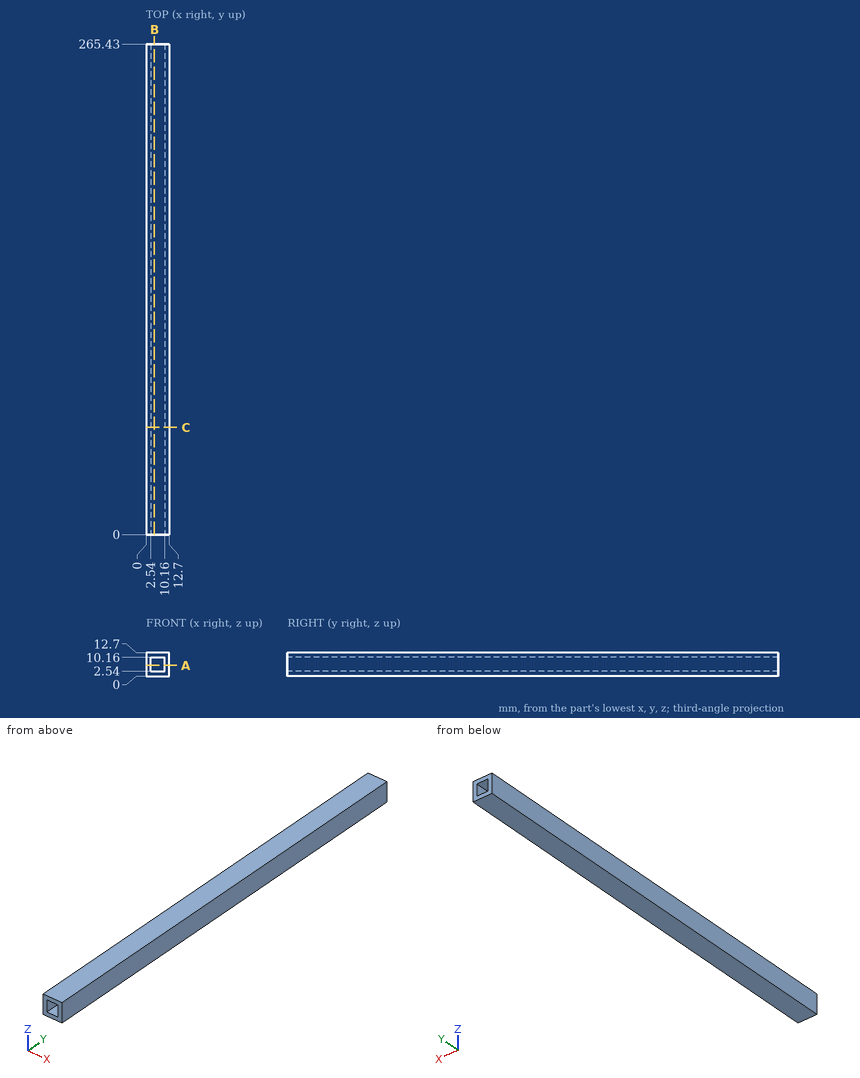
The drawing under review shows one solid part. Ordinate dimensions are in mm from its lowest x, y, z. Coordinates: 2 decimals unless noted, no trailing zeros. Order: outer loops, then holes, each group sorted by start corner. A loop starts at its lowest first (then second) coordinate and runs counter-clockwise, first axis right, second up. Notation, with made-up numbers: (45.5, -19) -> (71.5, -19) arc R19 ccw to (71.5, 13) -> close; hole circle Ø11 at (50, 9). An arc over 180 degrees is marked (long way). Answer in a Markdown table with one row per item. Add a question column.
Item 1: We need section A-A on z = 5.75. Write out the cut boundary in (x, y).
Item 2: We need section C-C on y = 58. Write out the cut boundary in (x, z), plus the area to 3 significant figures.
Item 3: To check wall thickness, follow probe 1 along X at (y, z) = (126, 7.75). State the ranges of the line that lie inside material, in increasing order.
Item 4: We need section B-B on x = 4.5. Write out the cut boundary in (y, z), plus the area to 3 significant figures.
Final values:
| question | item | result |
|---|---|---|
| 1 | outline | (0, 0) -> (2.54, 0) -> (2.54, 265.43) -> (0, 265.43) -> close; (10.16, 0) -> (12.7, 0) -> (12.7, 265.43) -> (10.16, 265.43) -> close |
| 2 | outline | (0, 0) -> (12.7, 0) -> (12.7, 12.7) -> (0, 12.7) -> close; hole (2.54, 2.54) -> (10.16, 2.54) -> (10.16, 10.16) -> (2.54, 10.16) -> close |
| 2 | area | 103 mm2 |
| 3 | probe 1 | x = 0 to 2.54, 10.16 to 12.7 |
| 4 | outline | (0, 0) -> (265.43, 0) -> (265.43, 2.54) -> (0, 2.54) -> close; (0, 10.16) -> (265.43, 10.16) -> (265.43, 12.7) -> (0, 12.7) -> close |
| 4 | area | 1,350 mm2 |
